Input: part model. Units: mm. Frame: model coordinates. A direction names the side the tool comes from. Coordinates: 2 decimals unless noted, no trailing zeros. Order: outer loops, then holes, each group sorted by start corner. A loop starts at its lowest first (then second) coordinate and runs counter-clockwise, first axis right, second up. Notation, with made-up numbers: (-32.75, 49.5) -> (-26.75, 49.5) arc R18 ccw to (-26.75, 78.5) -> close; hole circle Ø4 at (29, 60). An arc over 180 degrees is marked (long way). Answer as CSV lines item,"result".
from build123d import *

# Parameters (mm, degrees)
F3_W          = 50.8
F3_H          = 50.8
F3_W_2        = 47.498
F3_H_2        = 47.498
F4_DEPTH      = 25.4
F4_DEPTH_BACK = 787.4
F0_W          = 1524
F0_H          = 762
F0_W_2        = 1422.4
F0_H_2        = 660.4
F5_DEPTH      = 63.5
F6_R          = 1.651
F7_R          = 1.651


with BuildPart() as f4:
    # F3 (on line) → F4 (new body, two sides)
    with BuildSketch(Plane(origin=(-457.2, 0, -457.2), x_dir=(0.7071067812, 0, -0.7071067812), z_dir=(0.7071067812, 0, 0.7071067812))) as f4_sk:
        with Locations((-359.2102448428, 0)):
            Rectangle(F3_W, F3_H)
        with Locations((-359.2102448428, 0)):
            Rectangle(F3_W_2, F3_H_2, mode=Mode.SUBTRACT)
    extrude(amount=-F4_DEPTH)
    extrude(f4_sk.sketch, amount=F4_DEPTH_BACK)

    # F0 (on Front) → F5 (cut, symmetric)
    with BuildSketch(Plane.XZ):
        Rectangle(F0_W, F0_H)
        Rectangle(F0_W_2, F0_H_2, mode=Mode.SUBTRACT)
    extrude(amount=F5_DEPTH, both=True, mode=Mode.SUBTRACT)

    # F6
    f6_edges = [f4.edges().sort_by_distance(p)[0] for p in [
        (-462.460512, -25.4, 81.460512),
        (-462.460512, 25.4, 81.460512),
        (-426.539488, 25.4, 45.539488),
        (-426.539488, -25.4, 45.539488),
    ]]
    fillet(f6_edges, radius=F6_R)

    # F7
    f7_edges = [f4.edges().sort_by_distance(p)[0] for p in [
        (-427.706921, 23.749, 46.706921),
        (-427.706921, -23.749, 46.706921),
        (-461.293079, -23.749, 80.293079),
        (-461.293079, 23.749, 80.293079),
    ]]
    fillet(f7_edges, radius=F7_R)


solid = f4.part
1. Reachability of faces 5 (the face through (-181, 24, 330.2)), 6 (the face through (-449, -23.749, 60)) from +Z, -Z, +X, -X, +Y, -Y: full face, straight path, thin tool, end or side. Return the list, or none.
Findings:
face 5,"+Z, +X, -X, +Y, -Y"
face 6,"none"
2. Ray query, line 1 along Y through (x, z) = (-411, 106.5); line 2 along X through (y, z) = (2, 280); line 3 along X through (y, z) = (0.5, 31.5). Return the intervals inside material, ascending.
Findings:
line 1,"y = -25.4 to -23.75, 23.75 to 25.4"
line 2,"x = -263.92 to -261.59, -194.41 to -192.08"
line 3,"x = -512.42 to -510.09, -442.91 to -440.58"
3. Mould query, pull axis Z, two halves, no side actions, for faces 1 (the face through (-431.676, -0.309, 42.738)), 2 (the face through (-422.905, -24.929, 49.876)), 3 (the face through (-464.792, -0.309, 76.794)), 4 (the face through (-458.63, -24.9, 84.63)). Classes: released by +Z, released by -Z, zero draft, split by the parting line, or undercut.
Findings:
face 1,"undercut"
face 2,"released by -Z"
face 3,"undercut"
face 4,"released by +Z"
4. Cut plane A-A (y = -12.5). Return the cut outline in (x, z).
Findings:
outline,"(-711.2, -239.12) -> (-141.88, 330.2) -> (-144.21, 330.2) -> (-711.2, -236.79) -> close; (-711.2, -169.61) -> (-211.39, 330.2) -> (-213.72, 330.2) -> (-711.2, -167.28) -> close"
5. Contact query for flat-ended pins moving along their axis: pin 1 (1.5 mm diameter, centred on x = -440.5, y = 14, fed in from +Z); pin 2 (10 mm diameter, centred on y = 19, z = -63, fed in from +X); pin 3 (1.5 mm diameter, centred on y = -10, z = 232, fed in from -X); pin 4 (12 mm diameter, centred on x = -209.5, y = -15.5, fed in from +Z). Output: stop coordinate, or through.
Findings:
pin 1,"stops at z = 104.17"
pin 2,"stops at x = -530.08"
pin 3,"stops at x = -312.67"
pin 4,"stops at z = 330.2"
